Job drawing, mm, ordinate dimensions from the low corner. One solid piece. A direction names the side the tool comes from. Give positions to 0.01 mm unless a question says otherwise; leave off trailing zeros. Write each loop counter-clockwise with the first axis right and the second up, starting at its lowest first coordinate (ties: lowest second). Pieces come first, ordered by that corner, then holes. Notation, with made-up numbers: M 21,-31.5 L 63,-31.5 A15 ccw 63,-25.5 Z; hole C 10.5,10 d10. An arc over 180 degrees is marked long. Use CSV: the item, a comma, the result in double quotes. Start each with the question number.
Item 1: Drill centre lines: line 1 (Y direction, x = 3.5, z = 0.35) (3 decimals); line 2 (Y direction, x = 12, z = 1.4) (3 decimals); line 3 (X direction, y = 5, z = 1.95). Where is each one in solid material? Low to high. Write a range as [from, to].
Item 2: Which spindle directions (+Z, -Z, +X, -X, +Y, -Y) get a long thin tool onto all of the face, cutting with end or side? Do the marked faces 1, 2, 3, 4 and 5. Say none if no direction does.
Item 3: Cut at C-C (z = 0.65). List the corners of the cut face in (x, y) (3 decimals), then the cut area to 3 significant figures.
Item 4: Cut at A-A (x = 12). List the corners of the cut face in (y, z) (3 decimals), then the cut area to 3 significant figures.
Item 5: Cut at D-D (x = 47). List the corners of the cut face in (y, z).
Item 6: Pin check, flat tips, straight feed: pin 1 (1.9 mm diameter, centred on x = 8.5, z = 1, fed in from -Y); pin 2 (1.9 mm diameter, centred on x = 37.5, z = 2, fed in from +Y); pin 3 (1.9 mm diameter, centred on y = 42.5, z = 1.5, fed in from +X). Stop position of each tip, or through.
Item 7: Cut at B-B (y = 8). List the corners of the cut face in (x, z), then the cut area to 3 significant figures.
Item 8: Mould opens along X. For the marked faces 6, 7, 8 and 9 say: released by +X, released by -X, zero draft, split by the parting line, or undercut.
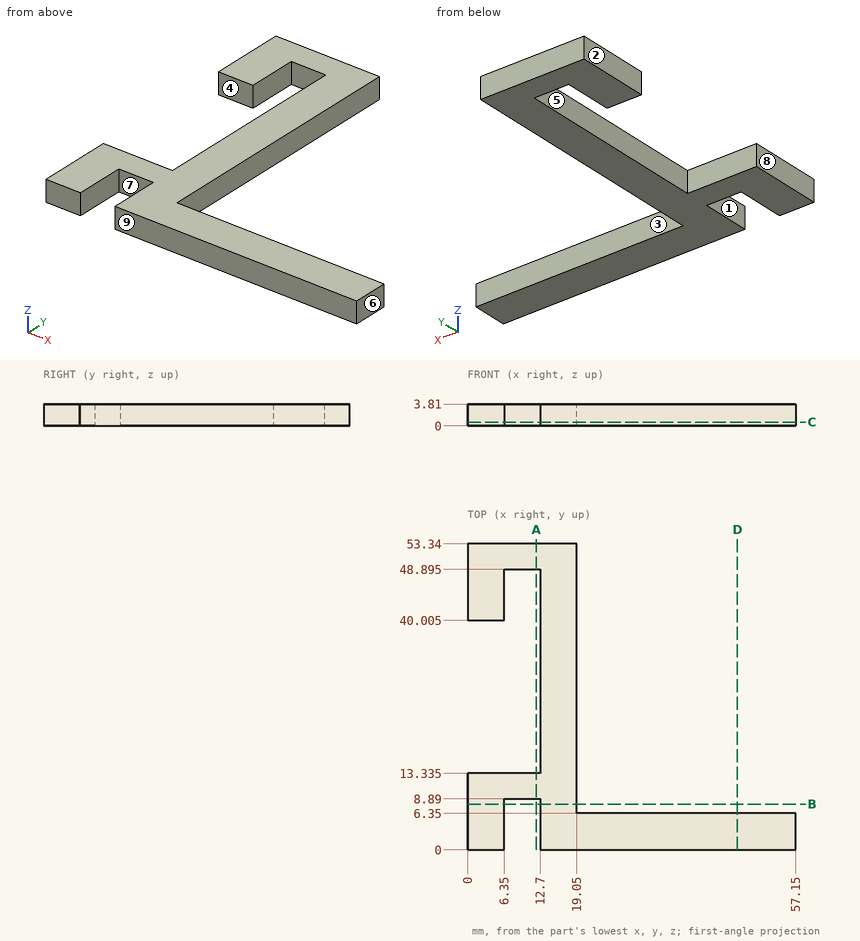
Worked answers:
1,line 1,"y = [0, 13.335], [40.005, 53.34]"
1,line 2,"y = [8.89, 13.335], [48.895, 53.34]"
1,line 3,"x = [0, 6.35], [12.7, 57.15]"
2,face 1,"+Z, -Z, -Y"
2,face 2,"+Z, -Z, -X, +Y, -Y"
2,face 3,"+Z, -Z, +X, +Y"
2,face 4,"+Z, -Z, -X"
2,face 5,"+Z, -Z"
3,outline,"M 0,0 L 6.35,0 L 6.35,8.89 L 12.7,8.89 L 12.7,0 L 57.15,0 L 57.15,6.35 L 19.05,6.35 L 19.05,53.34 L 0,53.34 L 0,40.005 L 6.35,40.005 L 6.35,48.895 L 12.7,48.895 L 12.7,13.335 L 0,13.335 Z"
3,area,"806 mm^2"
4,outline,"M 8.89,0 L 13.335,0 L 13.335,3.81 L 8.89,3.81 Z; M 48.895,0 L 53.34,0 L 53.34,3.81 L 48.895,3.81 Z"
4,area,"33.9 mm^2"
5,outline,"M 0,0 L 6.35,0 L 6.35,3.81 L 0,3.81 Z"
6,pin 1,"stops at y = 8.89"
6,pin 2,"stops at y = 6.35"
6,pin 3,"stops at x = 19.05"
7,outline,"M 0,0 L 6.35,0 L 6.35,3.81 L 0,3.81 Z; M 12.7,0 L 19.05,0 L 19.05,3.81 L 12.7,3.81 Z"
7,area,"48.4 mm^2"
8,face 6,"released by +X"
8,face 7,"undercut"
8,face 8,"released by -X"
8,face 9,"zero draft"
